Source: three-view drawing plus pictorial views. Frame: mm from the lowest corner of the part. A direction names the side the tool comes from. Round coordinates to 2 decimals unless told otherwise and drop trailing zeros. Loops run counter-clockwise (first coordinate to the right, second up) from the corner with the lowest first, then second, coordinate; pieces in that order, holes last. Notation, with made-up numbers: M -7,21 L 28,21 A26 cw 28,53 Z; hole C 32,40 d7. An arc over 180 degrees is marked long. Write each question's results on one line, items separated by ' | '.
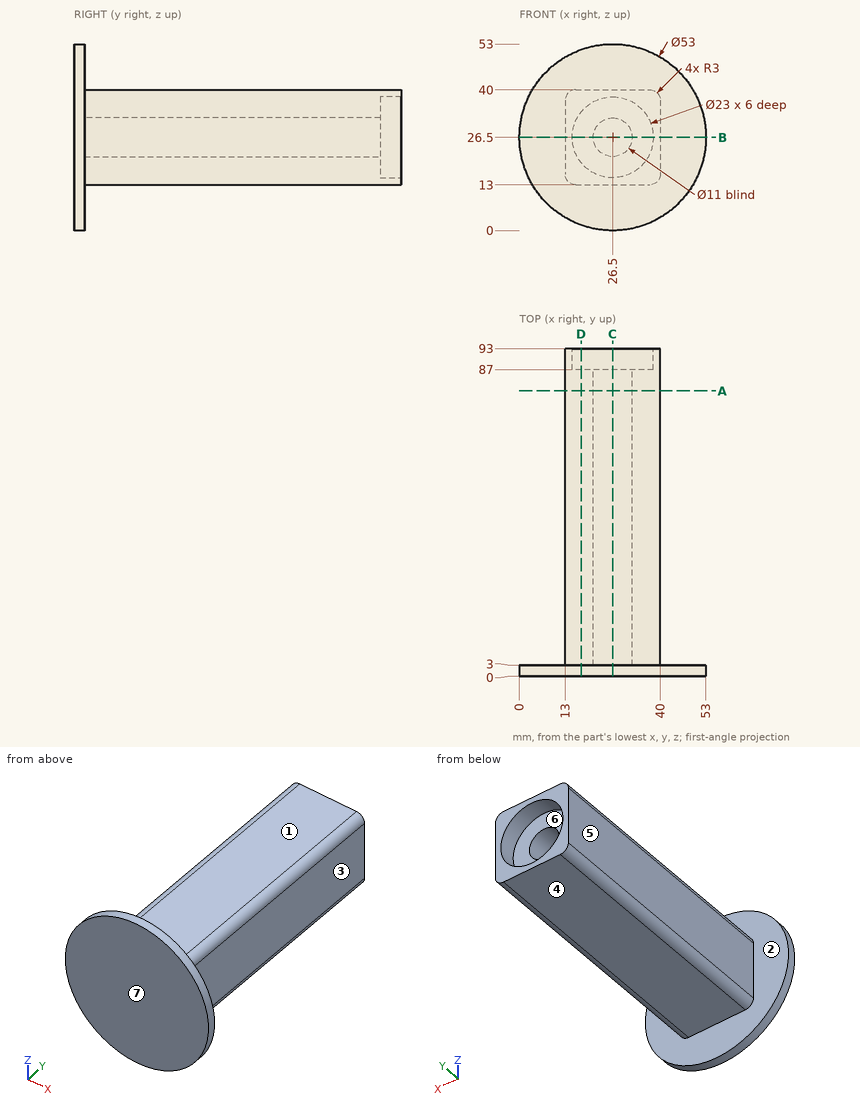
1. Section B-B (z = 26.5). Output: boundary loops of the cut face in (x, y), then the cut area to 3 significant figures.
Answer key:
outline: M 0,0 L 53,0 L 53,3 L 40,3 L 40,93 L 38,93 L 38,87 L 32,87 L 32,3 L 21,3 L 21,87 L 15,87 L 15,93 L 13,93 L 13,3 L 0,3 Z | area: 1,530 mm²
2. Pin query (flat end, axial travel): P1, Ø10, axis at x = 26.5, z = 26.5, coming from the +Y side; P2, Ø6.5, axis at y = 46.5, z = 26, coming from the +X side; P3, Ø6.5, axis at x = 30.5, y = 29.5, coming from the -Z side. Return the tip coordinate at first contact, or that it passes through.
Answer key:
P1: stops at y = 3 | P2: stops at x = 40 | P3: stops at z = 13
3. Section C-C (x = 26.5). Output: boundary loops of the cut face in (y, z).
Answer key:
outline: M 0,0 L 3,0 L 3,13 L 93,13 L 93,15 L 87,15 L 87,21 L 3,21 L 3,32 L 87,32 L 87,38 L 93,38 L 93,40 L 3,40 L 3,53 L 0,53 Z
4. Section D-D (x = 17.5). Output: boundary loops of the cut face in (y, z), then the cut area to 3 significant figures.
Answer key:
outline: M 0,1.58 L 3,1.58 L 3,13 L 93,13 L 93,19.34 L 87,19.34 L 87,33.66 L 93,33.66 L 93,40 L 3,40 L 3,51.42 L 0,51.42 Z | area: 2,490 mm²
5. Draft query along X for the marked faces 5, 6 and 7. Return one class per face: pulls with the +X half, pulls with the -X half, needs draft (parallel to the pull), parting line crosses it, or undercut.
Answer key:
face 5: pulls with the -X half | face 6: undercut | face 7: needs draft
6. Section A-A (y = 81). Output: boundary loops of the cut face in (x, z).
Answer key:
outline: M 13,16 A3 ccw 16,13 L 37,13 A3 ccw 40,16 L 40,37 A3 ccw 37,40 L 16,40 A3 ccw 13,37 Z; hole C 26.5,26.5 d11
7. Ray query, probe 1 along X at (y, z) = (70, 26); probe 2 along Z at (x, y) = (26, 90). Return the intervals inside material, ascending.
Answer key:
probe 1: x = 13 to 21.02, 31.98 to 40 | probe 2: z = 13 to 15.01, 37.99 to 40
8. Access query for the marked faces 1, 2, 3 and 4. Directions: +Z, -Z, +X, -X, +Y, -Y. A direction counts if a zero-diameter tool reaches every point of the face in a straight line with its end or side. Return the directions, or none.
Answer key:
face 1: +Z, +X, -X, +Y | face 2: +Y | face 3: +Z, -Z, +X, +Y | face 4: -Z, +X, -X, +Y
